The figure shows three views and two pictorial views of one solid part (mm, origin at its lowest corner). Answer the questions. Round coordinates to 2 decimals unless told otherwise and drop trailing zeros. Order: outer loops, then holes, each group sorted by start corner. A loop starts at its lowest first (then second) coordinate and runs counter-clockwise, first axis right, second up. Notation, with made-up numbers: (45, 78) - (60, 78) arc R19 cw to (60, 83) - close; hole circle Ø11 at (-15, 48). An arc over 180 degrees is marked (long way). Use CSV: the item, a comma, the result in double quotes.
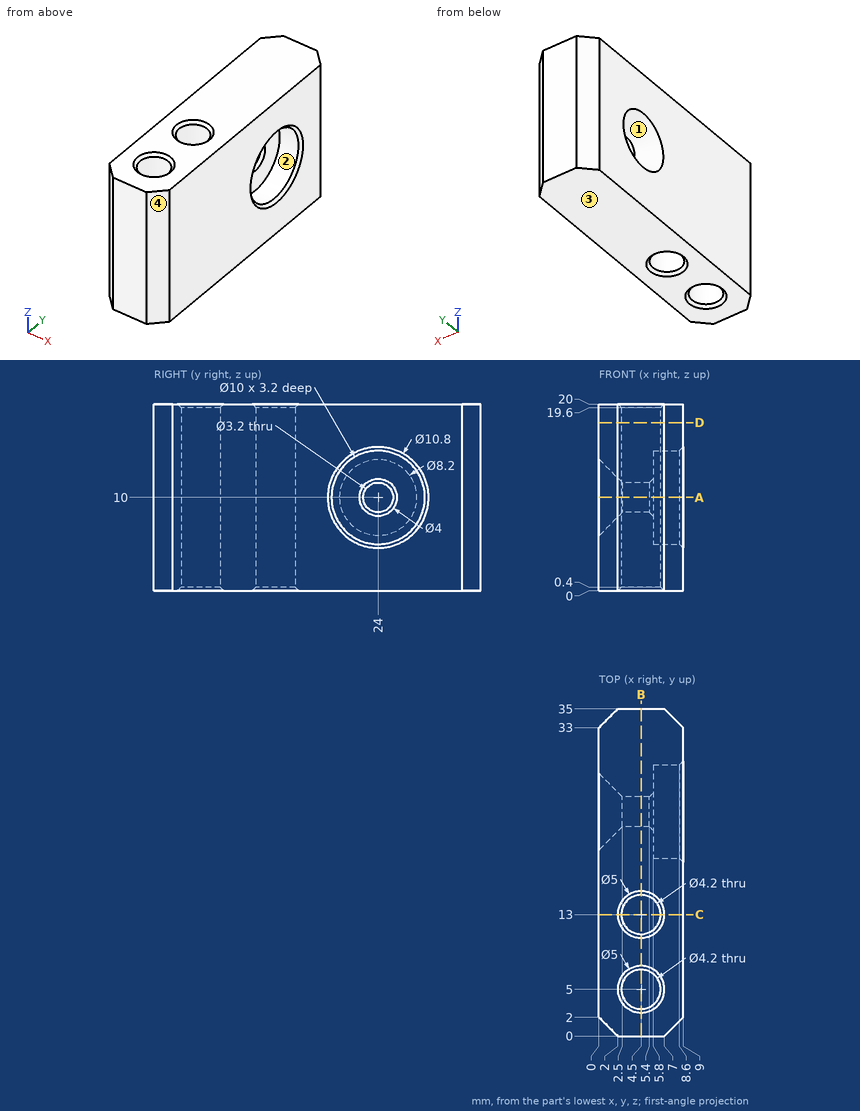
(1) The mould has two halves that part along Z. Classify the marked faces 1, 2, 3 and 4: released by +Z, released by -Z, zero draft, split by the parting line, or undercut.
Findings below:
face 1,"undercut"
face 2,"undercut"
face 3,"released by -Z"
face 4,"zero draft"
(2) Find section C-C (y = 13). Determine the outline of the cut face in (x, z).
Findings below:
outline,"(0, 0) - (2, 0) - (2.4, 0.4) - (2.4, 19.6) - (2, 20) - (0, 20) - close; (6.6, 0.4) - (7, 0) - (9, 0) - (9, 20) - (7, 20) - (6.6, 19.6) - close"
(3) Find section B-B (x = 4.5). Determine the outline of the cut face in (y, z), and give its area (3 significant figures).
Findings below:
outline,"(0, 0) - (2.5, 0) - (2.9, 0.4) - (2.9, 19.6) - (2.5, 20) - (0, 20) - close; (7.1, 0.4) - (7.5, 0) - (10.5, 0) - (10.9, 0.4) - (10.9, 19.6) - (10.5, 20) - (7.5, 20) - (7.1, 19.6) - close; (15.1, 0.4) - (15.5, 0) - (35, 0) - (35, 20) - (15.5, 20) - (15.1, 19.6) - close; hole circle Ø3.2 at (24, 10)"
area,"523 mm²"
(4) Find the intervals of material crossed by L1, parallel to Y at x = 3.25, z = 5; L2, parallel to Y at x = 4.5, z = 9.5; L3, parallel to Z at x = 3.7, y = 24, in increasing order. Write a range as from..to.
Findings below:
L1,"y = 0..3.31, 6.69..11.31, 14.69..35"
L2,"y = 0..2.9, 7.1..10.9, 15.1..22.48, 25.52..35"
L3,"z = 0..8.4, 11.6..20"
(5) Find section A-A (z = 10). Determine the outline of the cut face in (x, y).
Findings below:
outline,"(0, 2) - (2, 0) - (7, 0) - (9, 2) - (9, 18.6) - (8.6, 19) - (5.8, 19) - (5.8, 22) - (5.4, 22.4) - (2.5, 22.4) - (0, 19.9) - close; (0, 28.1) - (2.5, 25.6) - (5.4, 25.6) - (5.8, 26) - (5.8, 29) - (8.6, 29) - (9, 29.4) - (9, 33) - (7, 35) - (2, 35) - (0, 33) - close; hole circle Ø4.2 at (4.5, 5); hole circle Ø4.2 at (4.5, 13)"
(6) Find section D-D (z = 18). Determine the outline of the cut face in (x, y), and give its area (3 significant figures).
Findings below:
outline,"(0, 2) - (2, 0) - (7, 0) - (9, 2) - (9, 33) - (7, 35) - (2, 35) - (0, 33) - close; hole circle Ø4.2 at (4.5, 5); hole circle Ø4.2 at (4.5, 13)"
area,"279 mm²"
(7) Each of these flat-tipped pins is pushed along its axis until it touches: pin 1 (5 mm diameter, centred on y = 24, z = 10, fed in from +X); pin 2 (1 mm diameter, centred on x = 5.5, y = 5, fed in from -Z); pin 3 (6 mm diameter, centred on y = 24, z = 10, fed in from -X). Where does it stop, or does it pass through?
Findings below:
pin 1,"stops at x = 5.8"
pin 2,"passes through"
pin 3,"stops at x = 1.1"
